The listing builds one solid part. Answer for the finished solid, in the listing's coordinates (mm). Face numbers are marked on the shaded views. A direction names the side the tool comes from. Coordinates: 2 decimals unless noted, no trailing zeros. Order: outer loops, then holes, each group sorted by start corner. A loop starts at its lowest first (then second) coordinate and runs counter-clockwise, first axis right, second up.
```python
from build123d import *

# Parameters (mm, degrees)
F0_R     = 2.7
F1_DEPTH = 1.5
F2_W     = 120
F2_H     = 1.5
F3_DEPTH = 7.5
F4_R     = 5


with BuildPart() as f1:
    # F0 (on Front) → F1 (new body)
    with BuildSketch(Plane.XZ):
        with BuildLine():
            Line((-60, -71), (-60, -73.654599))
            ThreePointArc((-60, -73.654599), (0, -95), (60, -73.654599))
            Line((60, -73.654599), (60, -71))
            ThreePointArc((60, -71), (59.12132, -68.87868), (57, -68))
            Line((57, -68), (43.67577, -68))
            ThreePointArc((43.67577, -68), (40.225693, -68.614002), (37.199286, -70.380607))
            Line((37.199286, -70.380607), (22.800714, -82.619393))
            ThreePointArc((22.800714, -82.619393), (19.774307, -84.385998), (16.32423, -85))
            Line((16.32423, -85), (0, -85))
            Line((0, -85), (-16.32423, -85))
            ThreePointArc((-16.32423, -85), (-19.774307, -84.385998), (-22.800714, -82.619393))
            Line((-22.800714, -82.619393), (-37.199286, -70.380607))
            ThreePointArc((-37.199286, -70.380607), (-40.225693, -68.614002), (-43.67577, -68))
            Line((-43.67577, -68), (-57, -68))
            ThreePointArc((-57, -68), (-59.12132, -68.87868), (-60, -71))
        make_face()
        with BuildLine():
            ThreePointArc((60, -73.654599), (0, -95), (-60, -73.654599))
            Line((-60, -73.654599), (-60, -102))
            Line((-60, -102), (60, -102))
            Line((60, -102), (60, -73.654599))
        make_face()
        with Locations((-50, -85)):
            Circle(F0_R, mode=Mode.SUBTRACT)
        with Locations((50, -85)):
            Circle(F0_R, mode=Mode.SUBTRACT)
    extrude(amount=F1_DEPTH)

    # F2 (on face) → F3 (join)
    with BuildSketch(Plane.XZ.offset(1.5)):
        with Locations((0, -101.25)):
            Rectangle(F2_W, F2_H)
    extrude(amount=-F3_DEPTH)

    # F4
    f4_edges = [f1.edges().sort_by_distance(p)[0] for p in [
        (60, 6, -101.25),
        (-60, 6, -101.25),
    ]]
    fillet(f4_edges, radius=F4_R)


solid = f1.part
```
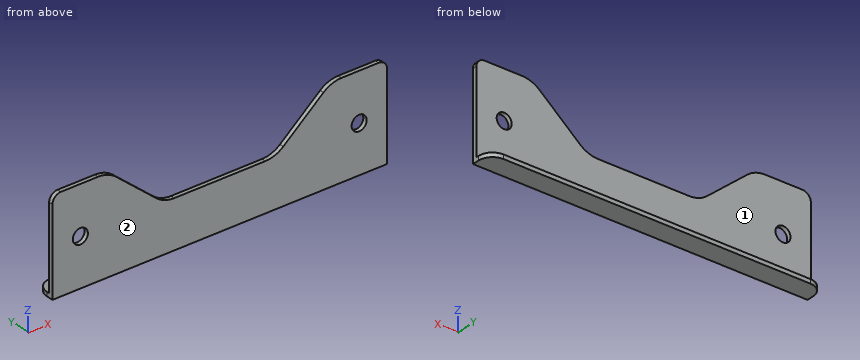
1) Each of these flat-tipped pins is pushed along its axis until it touches: P1, Ø8.5, axis at x = 50, z = -85, coming from the +Y side; P2, Ø1.6, axis at x = -3.5, y = -1, coming from the +Z side; P3, Ø1.8, axis at x = -7.5, y = 3.5, coming from the +Z side. Where does it stop, or does it pass through?
2) A cutting plane is placed at A-A, the plane x = -50. Write down the section's boundary in (y, z).
3) A cutting plane is placed at B-B, the plane x = 3. Write down the section's boundary in (y, z).
4) A cutting plane is placed at D-D, the plane x = 51.5. Write down the section's boundary in (y, z) (3 decimals), plus the area to 3 significant figures.
5) A cutting plane is placed at C-C, the plane z = -77. Write down the section's boundary in (x, y).
6) For the marked faces 1 and 2, determine the directions among +Z, -Z, +X, -X, +Y, -Y from which every point of the face is accessible in a straight line to the end or side of a thin tool.
7) Straight lines are drawn through the part: probe 1 along Z at (x, y) = (-50, -0.6); probe 2 along X at (y, z) = (-0.5, -83.5) (3 decimals); probe 3 along Y at (x, z) = (33.5, -89). For each, find the intervals that lie inside material, in ascending order.
Working result:
1. P1: stops at y = 0
1. P2: stops at z = -85
1. P3: stops at z = -100.5
2. outline: (-1.5, -102) - (6, -102) - (6, -100.5) - (0, -100.5) - (0, -87.7) - (-1.5, -87.7) - close; (-1.5, -82.3) - (0, -82.3) - (0, -68) - (-1.5, -68) - close
3. outline: (-1.5, -102) - (6, -102) - (6, -100.5) - (0, -100.5) - (0, -85) - (-1.5, -85) - close
4. outline: (-1.5, -102) - (6, -102) - (6, -100.5) - (0, -100.5) - (0, -87.245) - (-1.5, -87.245) - close; (-1.5, -82.755) - (0, -82.755) - (0, -68) - (-1.5, -68) - close
4. area: 53.3 mm2
5. outline: (-60, -1.5) - (-29.41, -1.5) - (-29.41, 0) - (-60, 0) - close; (29.41, -1.5) - (60, -1.5) - (60, 0) - (29.41, 0) - close
6. face 1: +Z, +X, -X, +Y
6. face 2: +Z, -Z, +X, -X, -Y
7. probe 1: z = -102 to -87.7, -82.3 to -68
7. probe 2: x = -60 to -52.245, -47.755 to -21.592, 21.592 to 47.755, 52.245 to 60
7. probe 3: y = -1.5 to 0
